Design review of the part shown in the three views and the two pictorial views. Dimensions are in mm from the part's minimum x, y and z. Coordinates: 2 decimals unless noted, no trailing zeros. Write each loop counter-clockwise with the first axis right and the second up, starting at its lowest first coordinate (ties: lowest second). Pieces come first, ordered by that corner, then holes. Notation, with made-up numbers: (58, -12) - (96, -12) arc R13 ccw to (96, -6) - close; hole circle Ø1 at (56, 49). An arc over 180 degrees is marked (long way). Return JSON: item names as keys, results as strings. Group by question number.
(1) Draft analysis for pull direction X (two halves, no side actions). For the marked faces 1, 2, 3 and 4, state which applies: released by +X, released by -X, zero draft, split by the parting line, or undercut.
(2) We need section C-C on y = 49. State the section outline as (x, z) points.
(3) We need section A-A on z = 27. Give the number of separate pieces and of enclosed holes in the cut face, then the cut area to 3 significant figures.
(4) We need section D-D on x = 28.5. State the section outline as (y, z) points, then the cut area to 3 significant figures.
(5) To check wall thickness, follow L1, parallel to X at y = 95, z = 15 (1 decimal); L2, parallel to X at y = 41.5, z = 15 (1 decimal); L3, parallel to X at y = 84, z = 18.5 (1 decimal). State the ranges of each line that lie inside material, in increasing order. Write a range as from..to.
(6) For pin 1 Ø1 at (x, z) = (109.5, 11) entering from -Y; pin 2 Ø12 at (y, z) = (54.5, 3) entering from -X; pin 3 Ø10 at (x, z) = (38, 16.5) entering from -Y, all flat-tipped, find the tip position at first contact; note any pin that passes through.
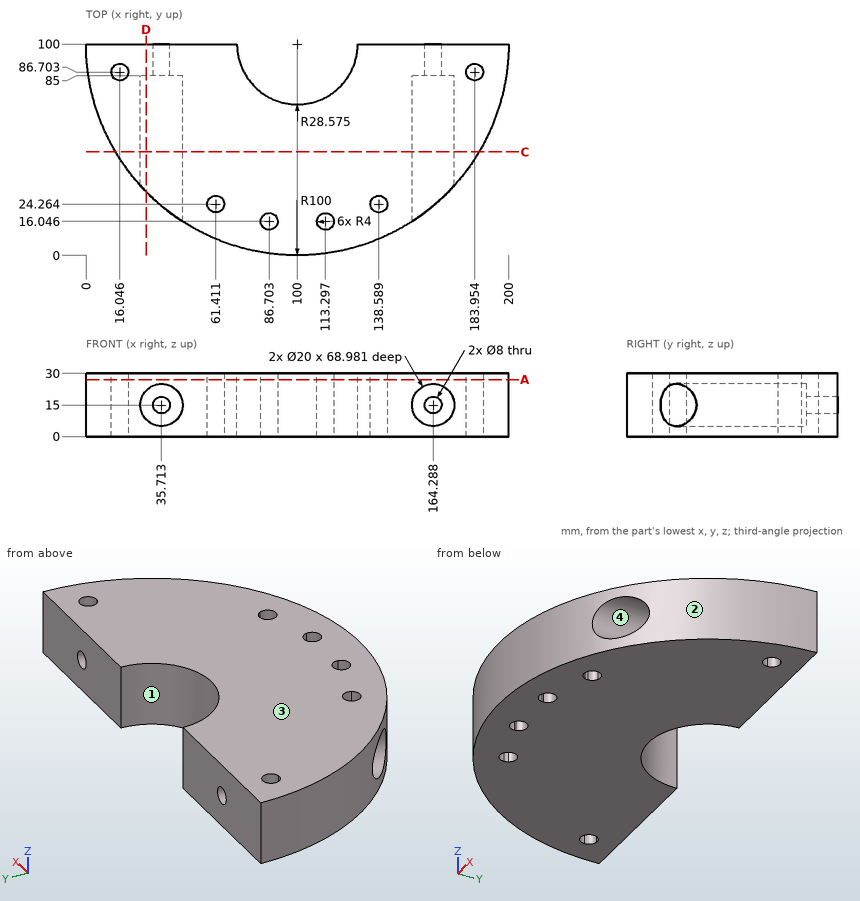
Ans:
{
 "1": {"face 1": "undercut", "face 2": "split by the parting line", "face 3": "zero draft", "face 4": "undercut"},
 "2": {"outline": "(13.98, 0) - (186.02, 0) - (186.02, 30) - (13.98, 30) - close; hole circle Ø20 at (35.71, 15); hole circle Ø20 at (164.29, 15)"},
 "3": {"separate pieces": "1", "enclosed holes": "6", "area": "14,100 mm²"},
 "4": {"outline": "(30.09, 0) - (100, 0) - (100, 30) - (30.09, 30) - (30.09, 21.93) - (85, 21.93) - (85, 8.07) - (30.09, 8.07) - close", "area": "1,340 mm²"},
 "5": {"L1": "0.1..31.7, 39.7..71.9, 128.1..160.3, 168.3..199.9", "L2": "18.9..25.7, 45.7..154.3, 174.3..181.1", "L3": "1.3..13.1, 19..26.3, 45.1..76.3, 123.7..154.9, 173.7..181, 186.9..198.7"},
 "6": {"pin 1": "y = 0.41", "pin 2": "x = 8.13", "pin 3": "y = 85"}
}
